```python
from build123d import *

# Parameters (mm, degrees)
F0_W     = 30
F0_H     = 30
F0_R     = 10.31875
F1_DEPTH = 3.96875
F0_W_2   = 115
F2_DEPTH = 15


# Not quite as in the source:
# - a length typed as a fraction of an inch, garbled in the dataset ("3 / 203.2 mm" for 3/8 in), is restored


with BuildPart() as f1:
    # F0 (on Right) → F1 (new body, symmetric)
    with BuildSketch(Plane.YZ):
        Rectangle(F0_W, F0_H)
        Circle(F0_R, mode=Mode.SUBTRACT)
    extrude(amount=F1_DEPTH, both=True)

    # F0 (on Right) → F2 (join, symmetric)
    with BuildSketch(Plane.YZ):
        with Locations((72.5, 0)):
            Rectangle(F0_W_2, F0_H)
    extrude(amount=F2_DEPTH, both=True)


solid = f1.part
```
Geometry: final body of the model. Coordinates: model frame, mm. A direction names the side the tool comes from. Give positions to 0.01 mm unless a question says otherwise; leave off trailing zeros. Write each loop counter-clockwise with the first axis right and the second up, starting at its lowest first coordinate (ties: lowest second). Pieces come first, ordered by that corner, then holes.
1. Draft query along Y for faces 4 (the flat face through (-9, 15, 0)), 5 (the cylindrical face through (-0.056, -2.237, -10.073)), 6 (the flat face through (0, 73, -15)), 7 (the flat face through (0, 130, 0)). Return one class per face: released by +Y, released by -Y, zero draft, split by the parting line, or undercut.
2. Line query: probe 1 along Z at (x, y) = (-1.25, 0); probe 2 along Y at (x, z) = (-10.5, -13); probe 3 along Y at (x, z) = (-3.25, 9). Output: solid intervals per line, ascending.
3. Section query A-A, the plane y = 0. Return loops of the section in (x, z).
4. Section query B-B, the plane z = 0. Return loops of the section in (x, y), then the cut area to 3 significant figures.
5. Pin query (flat end, axial travel): P1, Ø15, axis at y = 1, z = -6, coming from the +X side; P2, Ø3.5, axis at x = -8, z = -4, coming from the -Y side. Return the tip coordinate at first contact, or that it passes through.
6. Reachability of faces 1 (the flat face through (0, 73, 15)), 2 (the flat face through (-3.969, -4, 10)), 3 (the flat face through (10, 15, 0)) from +Z, -Z, +X, -X, +Y, -Y: full face, straight path, thin tool, end or side. Return the list, or none.
7. Section query C-C, the plane z = 13. Return loops of the section in (x, y), then the cut area to 3 significant figures.
8. Section query D-D, the plane x = -0.5. Return loops of the section in (y, z), then the cut area to 3 significant figures.
Computed:
1. face 4: released by -Y
1. face 5: undercut
1. face 6: zero draft
1. face 7: released by +Y
2. probe 1: z = -15 to -10.32, 10.32 to 15
2. probe 2: y = 15 to 130
2. probe 3: y = -15 to -5.05, 5.05 to 130
3. outline: (-3.97, -15) - (3.97, -15) - (3.97, -10.32) - (-3.97, -10.32) - close; (-3.97, 10.32) - (3.97, 10.32) - (3.97, 15) - (-3.97, 15) - close
4. outline: (-15, 15) - (-3.97, 15) - (-3.97, 10.32) - (3.97, 10.32) - (3.97, 15) - (15, 15) - (15, 130) - (-15, 130) - close; (-3.97, -15) - (3.97, -15) - (3.97, -10.32) - (-3.97, -10.32) - close
4. area: 3,520 mm2
5. P1: stops at x = 3.97
5. P2: stops at y = 15
6. face 1: +Z, +X, -X, +Y, -Y
6. face 2: +Z, -Z, -X, -Y
6. face 3: +Z, -Z, +X, -Y
7. outline: (-15, 15) - (-3.97, 15) - (-3.97, -15) - (3.97, -15) - (3.97, 15) - (15, 15) - (15, 130) - (-15, 130) - close
7. area: 3,690 mm2
8. outline: (-15, -15) - (130, -15) - (130, 15) - (-15, 15) - close; hole circle Ø20.64 at (0, 0)
8. area: 4,020 mm2
